CAD build for the part. Positions are in the model's coordinates, mm. A direction names the side the tool comes from. Give positions to 0.01 mm unless a question says otherwise; leave off trailing zeros. Order: outer loops, then holes, each group sorted by start corner. A loop starts at its lowest first (then second) coordinate and runs counter-clockwise, first axis right, second up. Notation, with made-up numbers: M 57,24.5 L 94,24.5 A19 ccw 94,61.5 Z; hole C -17,47.25 d8. An arc over 180 degrees is marked long. Put each result on its own line as item: value. Start each with the question number.
1) Drill centre lines: line 1 (Y direction, x = 3.5, z = 56); line 2 (X direction, y = -30.5, z = 60); line 3 (Z direction, x = 42, y = -55.5). Where is each one in solid material? Low to high. Write a range as [from, to].
2) Cut at D-D (y = -35). Write the cut outline in (x, z).
3) Cut at C-C (z = 25). Write the cut outline in (x, y), and give its area (3 significant figures).
4) Pin check, flat tips, straight feed: pin 1 (10 mm diameter, centred on y = -45.5, z = -5.5, fed in from -X); pin 2 (17 mm diameter, centred on x = 22.5, z = 47.5, fed in from -Y); pin 3 (1.5 mm diameter, centred on x = 51.5, y = -14.5, fed in from +Z). Stop position of each tip, or through.
5) Two-plate mould, pull along Z, no slides. Class faces 3 (the face through (21, -30, 38)), 4 (the face through (74.816, -30, 33)), 5 (the face through (-15.165, -1.424, 73.563)), 6 (the face through (24.47, -2.54, -14.29)): released by +Z, released by -Z, zero draft, split by the parting line, or undercut.
6) Cut at B-B (x = 39). Write the cut outline in (y, z), and give its area (3 significant figures).
7) Cut at A-A (y = -27). Write the cut outline in (x, z).
8) Tool access for faces 1 (the face through (24, -30, -16.752)), 2 (the face through (0.139, -45.21, 57.065)): list every direction of +Z, -Z, +X, -X, +Y, -Y with a clear straight run to the whole face (end or side of a thin tool).
```python
from build123d import *

# Parameters (mm, degrees)
F1_DEPTH = 60
F2_R     = 5
F3_SIZE  = 5
F4_R     = 28.16198
F5_DEPTH = 30


with BuildPart() as f1:
    # F0 (on Front) → F1 (new body)
    with BuildSketch(Plane.XZ):
        with BuildLine():
            Line((49.816129, 83.248417), (-0.183871, 83.248417))
            ThreePointArc((-0.183871, 83.248417), (-17.861541, 75.926086), (-25.183871, 58.248417))
            Line((-25.183871, 58.248417), (-25.183871, 8.248417))
            ThreePointArc((-25.183871, 8.248417), (-17.861541, -9.429253), (-0.183871, -16.751583))
            Line((-0.183871, -16.751583), (49.816129, -16.751583))
            ThreePointArc((49.816129, -16.751583), (67.493798, -9.429253), (74.816129, 8.248417))
            Line((74.816129, 8.248417), (74.816129, 58.248417))
            ThreePointArc((74.816129, 58.248417), (67.493798, 75.926086), (49.816129, 83.248417))
        make_face()
    extrude(amount=F1_DEPTH)

    # F2
    f2_edges = [f1.edges().sort_by_distance(p)[0] for p in [
        (74.816129, -60, 33.248417),
        (67.493798, -60, 75.926086),
        (24.816129, -60, 83.248417),
        (-17.861541, -60, 75.926086),
        (-25.183871, -60, 33.248417),
        (-17.861541, -60, -9.429253),
        (24.816129, -60, -16.751583),
        (67.493798, -60, -9.429253),
    ]]
    fillet(f2_edges, radius=F2_R)

    # F3
    f3_edges = [f1.edges().sort_by_distance(p)[0] for p in [
        (74.816129, 0, 33.248417),
        (67.493798, 0, 75.926086),
        (24.816129, 0, 83.248417),
        (-17.861541, 0, 75.926086),
        (-25.183871, 0, 33.248417),
        (-17.861541, 0, -9.429253),
        (24.816129, 0, -16.751583),
        (67.493798, 0, -9.429253),
    ]]
    chamfer(f3_edges, length=F3_SIZE)

    # F4 (on face) → F5 (cut)
    with BuildSketch(Plane.XZ.offset(60)):
        with Locations((20.895224, 38.032025)):
            Circle(F4_R)
    extrude(amount=-F5_DEPTH, mode=Mode.SUBTRACT)


solid = f1.part
```
Solution:
1. line 1: [-30, 0]
1. line 2: [-25.12, 3.27], [38.52, 74.75]
1. line 3: [-16.73, 19.39], [56.68, 83.22]
2. outline: M -25.18,8.25 A25 ccw -0.18,-16.75 L 49.82,-16.75 A25 ccw 74.82,8.25 L 74.82,58.25 A25 ccw 49.82,83.25 L -0.18,83.25 A25 ccw -25.18,58.25 Z; hole C 20.9,38.03 d56.32
3. outline: M -25.18,-55 A5 ccw -20.18,-60 L -4.07,-60 L -4.07,-30 L 45.86,-30 L 45.86,-60 L 69.82,-60 A5 ccw 74.82,-55 L 74.82,-5 L 69.82,0 L -20.18,0 L -25.18,-5 Z
3. area: 4,470 mm²
4. pin 1: x = -23.6
4. pin 2: y = -30
4. pin 3: z = 83.23
5. face 3: undercut
5. face 4: zero draft
5. face 5: released by +Z
5. face 6: released by -Z
6. outline: M -60,-11.75 A5 ccw -55,-16.75 L -5,-16.75 L 0,-11.75 L 0,78.25 L -5,83.25 L -55,83.25 A5 ccw -60,78.25 L -60,59.6 L -30,59.6 L -30,16.46 L -60,16.46 Z
6. area: 4,670 mm²
7. outline: M -25.18,8.25 A25 ccw -0.18,-16.75 L 49.82,-16.75 A25 ccw 74.82,8.25 L 74.82,58.25 A25 ccw 49.82,83.25 L -0.18,83.25 A25 ccw -25.18,58.25 Z
8. face 1: -Z, +X, -X, +Y, -Y
8. face 2: -Y
